The listing builds one solid part. Answer for the finished solid, in the listing's coordinates (mm). A direction names the side the tool comes from. Give positions to 0.01 mm unless a question says otherwise; leave off trailing zeros. Loops run counter-clockwise (first coordinate to the right, second up) from the corner with the lowest first, then second, coordinate; pieces in that order, holes last.
Item 1: Consider line 1 along X through (y, z) = (6.5, 0); line 2 along X through (y, z) = (22, 0); line 3 along Y through (x, z) = (6, -41.5). Determine where each line is inside the solid, lowest interval first.
Item 2: Section C-C, the plane z = -36 is taken. Give the vertices of the cut face in (x, y).
Item 3: Section B-B, the plane z = 0 is taken. Give the vertices of the cut face in (x, y), and give its area (3 significant figures).
Item 4: Section D-D, the plane x = 43 is taken. Give the vertices of the cut face in (y, z).
Item 5: Section A-A, the plane x = 0 is taken. Give the vertices of the cut face in (y, z), and give its area (3 significant figures).
Item 6: A tool of negligible diameter and unlimited length cuts with its end or side. For faces 1 (the face through (-52.3, 5, 39.9)), 2 (the face through (-2.06, 18.49, 54.96)), 3 (the face through (-57.287, 2.465, 31.353)), from which of +Z, -Z, +X, -X, +Y, -Y can it reach the whole face along a straight path? Write none if from no direction.
Item 7: The mould has two halves that part along X. Classify faces 4 (the face through (0, 7.5, 48)), 5 (the face through (-57.4, 2.465, -30.606)), 6 (the face through (-53, 5, -37)): pulls with the +X half, pulls with the -X half, needs draft (parallel to the pull), parting line crosses it, or undercut.
Item 8: Each of these flat-tipped pins is pushed along its axis until it touches: pin 1 Ø12 at (x, y) = (32.5, 22) entering from -Z; pin 2 Ø1.5 at (x, y) = (-28.5, 9.5) entering from -Z; pin 3 Ø12 at (x, z) = (16.5, -2) entering from +Y; pin 4 Ø5 at (x, z) = (50.28, -37.07) entering from -Y. Where does it stop, or does it pass through?
from build123d import *

# Parameters (mm, degrees)
SKETCH_1_R          = 55
EXTRUDE_1_DEPTH     = 37.5
SKETCH_3_R          = 49.5
CUT_EXTRUDE_1_DEPTH = 32.5
SKETCH_5_W          = 43
SKETCH_5_H          = 12.242897151
CUT_EXTRUDE_2_DEPTH = 40
FILLET_4_R          = 2
FILLET_5_R          = 2
SKETCH_6_R          = 6.65
CUT_EXTRUDE_3_DEPTH = 12
EXTRUDE_START       = -5
EXTRUDE_3_DEPTH     = 5
FILLET_7_R          = 10
FILLET_8_R          = 5
SKETCH_10_R         = 3
CUT_EXTRUDE_5_DEPTH = 5
EXTRUDE_START_2     = 2.5
EXTRUDE_4_DEPTH     = 2.5


with BuildPart() as part:
    # 草图1 → 凸台-拉伸1 (new body)
    with BuildSketch(Plane(origin=(0, 0, 0), x_dir=(1, 0, 0), z_dir=(0, 1, 0))):
        with Locations(Location((0, 0, 0), (0, 0, 270))):
            Circle(SKETCH_1_R)
    extrude(amount=EXTRUDE_1_DEPTH)

    # 草图3 → 切除-拉伸1 (cut)
    with BuildSketch(Plane(origin=(0, 37.5, 0), x_dir=(1, 0, 0), z_dir=(0, 1, 0))):
        with Locations(Location((0, 0, 0), (0, 0, 270))):
            Circle(SKETCH_3_R)
    extrude(amount=-CUT_EXTRUDE_1_DEPTH, mode=Mode.SUBTRACT)

    # 草图5 → 切除-拉伸2 (cut)
    with BuildSketch(Plane(origin=(0, 37.5, 0), x_dir=(1, 0, 0), z_dir=(0, 1, 0))):
        with Locations((0, 50.708442195)):
            Rectangle(SKETCH_5_W, SKETCH_5_H)
    extrude(amount=-CUT_EXTRUDE_2_DEPTH, mode=Mode.SUBTRACT)

    # 圆角4
    fillet_4_edges = [part.edges().sort_by_distance(p)[0] for p in [
        (-21.5, 18.75, -50.623611092),
    ]]
    fillet(fillet_4_edges, radius=FILLET_4_R)

    # 圆角5
    fillet_5_edges = [part.edges().sort_by_distance(p)[0] for p in [
        (21.5, 18.75, -50.623611092),
    ]]
    fillet(fillet_5_edges, radius=FILLET_5_R)

    # 草图6 → 切除-拉伸3 (cut)
    with BuildSketch(Plane(origin=(0, 5, 0), x_dir=(1, 0, 0), z_dir=(0, 1, 0))):
        with Locations(Location((0, 0, 0), (0, 0, 270))):
            Circle(SKETCH_6_R)
    extrude(amount=-CUT_EXTRUDE_3_DEPTH, mode=Mode.SUBTRACT)

    # 草图14 → 凸台-拉伸3 (add)
    with BuildSketch(Plane(origin=(0, 5, 0), x_dir=(1, 0, 0), z_dir=(0, 1, 0)).offset(EXTRUDE_START)):
        with BuildLine():
            Line((-49.898576095, 23.132922507), (-63.862525635, 37.044772973))
            Line((-63.862525635, 37.044772973), (-49.746845912, 51.213315099))
            Line((-49.746845912, 51.213315099), (-38.128637352, 39.638453724))
            ThreePointArc((-38.128637352, 39.638453724), (-44.78063998, 31.932652301), (-49.898576095, 23.132922507))
        make_face()
        with BuildLine():
            Line((49.811900188, -23.3189751), (64.421720913, -37.928795825))
            Line((64.421720913, -37.928795825), (50.279585289, -52.070931449))
            Line((50.279585289, -52.070931449), (37.984884655, -39.776230814))
            ThreePointArc((37.984884655, -39.776230814), (44.662950793, -32.097053236), (49.811900188, -23.3189751))
        make_face()
        with BuildLine():
            Line((-49.632393674, -23.698639164), (-63.862550335, -37.928795825))
            Line((-63.862550335, -37.928795825), (-49.720414711, -52.070931449))
            Line((-49.720414711, -52.070931449), (-37.697852746, -40.048369484))
            ThreePointArc((-37.697852746, -40.048369484), (-44.423770724, -32.427281642), (-49.632393674, -23.698639164))
        make_face()
        with BuildLine():
            Line((38.475737251, 39.301623923), (50.118901666, 51.212426922))
            Line((50.118901666, 51.212426922), (64.420808036, 37.231887798))
            Line((64.420808036, 37.231887798), (50.134465219, 22.6171483))
            ThreePointArc((50.134465219, 22.6171483), (45.083643676, 31.50341367), (38.475737251, 39.301623923))
        make_face()
    extrude(amount=EXTRUDE_3_DEPTH)

    # 圆角7
    fillet_7_edges = [part.edges().sort_by_distance(p)[0] for p in [
        (-38.128637352, 2.5, -39.638453724),
        (-49.898576095, 2.5, -23.132922507),
        (-49.632393674, 2.5, 23.698639164),
        (-37.697852746, 2.5, 40.048369484),
        (50.134465219, 2.5, -22.6171483),
        (38.475737251, 2.5, -39.301623923),
        (37.984884655, 2.5, 39.776230814),
        (49.811900188, 2.5, 23.3189751),
    ]]
    fillet(fillet_7_edges, radius=FILLET_7_R)

    # 圆角8
    fillet_8_edges = [part.edges().sort_by_distance(p)[0] for p in [
        (-63.862525635, 2.5, -37.044772973),
        (-49.746845912, 2.5, -51.213315099),
        (-49.720414711, 2.5, 52.070931449),
        (-63.862550335, 2.5, 37.928795825),
        (50.118901666, 2.5, -51.212426922),
        (64.420808036, 2.5, -37.231887798),
        (50.279585289, 2.5, 52.070931449),
        (64.421720913, 2.5, 37.928795825),
    ]]
    fillet(fillet_8_edges, radius=FILLET_8_R)

    # 草图10 → 切除-拉伸5 (cut)
    with BuildSketch(Plane(origin=(0, 5, 0), x_dir=(1, 0, 0), z_dir=(0, 1, 0))):
        with Locations(Location((-49.720414711, 37.071204175, 0), (0, 0, 270))):
            Circle(SKETCH_10_R)
        with Locations(Location((50.279585289, 37.071204175, 0), (0, 0, 270))):
            Circle(SKETCH_10_R)
        with Locations(Location((-49.720414711, -37.928795825, 0), (0, 0, 270))):
            Circle(SKETCH_10_R)
        with Locations(Location((50.279585289, -37.928795825, 0), (0, 0, 270))):
            Circle(SKETCH_10_R)
    extrude(amount=-CUT_EXTRUDE_5_DEPTH, mode=Mode.SUBTRACT)

    # 草图15 → 凸台-拉伸4 (add)
    with BuildSketch(Plane(origin=(0, 5, 0), x_dir=(1, 0, 0), z_dir=(0, 1, 0)).offset(EXTRUDE_START_2)):
        with BuildLine():
            Line((-21.5, 44.586993619), (-16.255768207, 44.586993619))
            ThreePointArc((-16.255768207, 44.586993619), (0, -47.457876059), (16.255768207, 44.586993619))
            Line((16.255768207, 44.586993619), (21.5, 44.586993619))
            ThreePointArc((21.5, 44.586993619), (0, -49.5), (-21.5, 44.586993619))
        make_face()
    extrude(amount=-EXTRUDE_4_DEPTH)


solid = part.part
Worked answers:
1. line 1: x = -55 to -47.46, 47.46 to 55
1. line 2: x = -55 to -49.5, 49.5 to 55
1. line 3: y = 0 to 5
2. outline: (-61.68, 0) - (-52.52, 0) - (-52.52, 5) - (-61.68, 5) - close; (-46.92, 0) - (47.48, 0) - (47.48, 5) - (41.58, 5) - (41.58, 37.5) - (33.97, 37.5) - (33.97, 7.5) - (30.92, 7.5) - (30.92, 5) - (-30.92, 5) - (-30.92, 7.5) - (-33.97, 7.5) - (-33.97, 37.5) - (-41.58, 37.5) - (-41.58, 5) - (-46.92, 5) - close; (53.08, 0) - (62.22, 0) - (62.22, 5) - (53.08, 5) - close
3. outline: (-55, 0) - (-6.65, 0) - (-6.65, 5) - (-47.46, 5) - (-47.46, 7.5) - (-49.5, 7.5) - (-49.5, 37.5) - (-55, 37.5) - close; (6.65, 0) - (55, 0) - (55, 37.5) - (49.5, 37.5) - (49.5, 7.5) - (47.46, 7.5) - (47.46, 5) - (6.65, 5) - close
3. area: 851 mm2
4. outline: (0, -44.37) - (5, -44.37) - (5, -34.29) - (37.5, -34.29) - (37.5, -24.52) - (7.5, -24.52) - (7.5, -20.08) - (5, -20.08) - (5, 20.08) - (7.5, 20.08) - (7.5, 24.52) - (37.5, 24.52) - (37.5, 34.29) - (5, 34.29) - (5, 45.02) - (0, 45.02) - close
5. outline: (0, -44.59) - (5, -44.59) - (5, -6.65) - (0, -6.65) - close; (0, 6.65) - (5, 6.65) - (5, 47.46) - (7.5, 47.46) - (7.5, 49.5) - (37.5, 49.5) - (37.5, 55) - (0, 55) - close
5. area: 615 mm2
6. face 1: +Z, -X, +Y
6. face 2: +Y
6. face 3: -X, +Y, -Y
7. face 4: undercut
7. face 5: pulls with the -X half
7. face 6: needs draft
8. pin 1: stops at z = -48.19
8. pin 2: stops at z = -47.49
8. pin 3: stops at y = 5
8. pin 4: passes through
